Source: CAD feature listing. Evaluate the final solid. Frame: model axes, mm. Face numbers are marked on the shaded views. A direction names the side the tool comes from. Round coordinates to 2 decimals unless told otherwise and drop trailing zeros. Loops run counter-clockwise (first coordinate to the right, second up) from the corner with the lowest first, then second, coordinate; pieces in that order, holes last.
(1) Material intervals for probe 1 along X at (y, z) = (-3.25, 0.75); probe 2 along Z at (x, y) = (1.5, 2.75); probe 3 along X at (y, z) = (2.75, 3.5), sorted ascending.
(2) Section C-C, the plane x = 0. Return the cut outline in (y, z).
(3) Mould query, pull axis X, two halves, no side actions, for the marked faces 4 and 5. Classes: pulls with the +X half, pulls with the -X half, needs draft (parallel to the pull), parting line crosses it, or undercut.
(4) First-contact query: pin 1 Ø1 at (x, z) = (2.5, -3.5) entering from -Y; pin 2 Ø1.8 at (x, y) = (-2.5, 1.5) entering from -Z; pin 3 Ø2 at (x, z) = (-1.5, -3.5) entering from -Y. Flat tips, straight axial feed; report the tip coordinate or a pass-through.
(5) Section B-B, the plane y = 0. Return the cut outline in (x, z).
(6) Set-up query: the marked faces 1, 2 and 3. Return all of +Z, -Z, +X, -X, +Y, -Y with unobstructed straight access to the full face (end or side cutting, diameter ignored); none if empty.
```python
from build123d import *
from build123d import SkipClean  # not in build123d's __all__

# Parameters (mm, degrees)
F1_DEPTH     = 5
F2_DEPTH     = 5
F3_T3_DEPTH  = 12.521557359
F3_T6_ANGLE  = 198.0325102457
F3_T9_ANGLE  = 198.0325102457
F3_T12_DEPTH = 12.521557359
F3_T15_ANGLE = 209.516708524
F3_T18_DEPTH = 12.571682988
F3_T21_ANGLE = 144.0077008654
F3_T24_ANGLE = 53.9966137912
F3_T27_DEPTH = 7.0466201735
F3_T31_DEPTH = 8.0466201735


# Not quite as in the source:
# - a fillet or chamfer that OpenCascade refuses, or shapes differently, is made with other operations: its cross-section is extruded or revolved along the edge and cut away or added


with BuildPart() as f1:
    # F0 (on Top) → F1 (new body)
    with BuildSketch(Plane.XY):
        with BuildLine():
            ThreePointArc((-3.5355339059, -3.5355339059), (-2.1422777427, -4.5178143026), (-0.5, -4.9749371855))
            Line((-0.5, -4.9749371855), (-0.5, -0.5))
            Line((-0.5, -0.5), (-3.5355339059, -3.5355339059))
        make_face()
        with BuildLine():
            ThreePointArc((-0.5, -4.9749371855), (-0.2503138753, -4.9937303656), (0, -5))
            Line((0, -5), (0, 0))
            Line((0, 0), (-0.5, -0.5))
            Line((-0.5, -0.5), (-0.5, -4.9749371855))
        make_face()
        with BuildLine():
            ThreePointArc((0, -5), (0.2503138753, -4.9937303656), (0.5, -4.9749371855))
            Line((0.5, -4.9749371855), (0.5, 0.5))
            Line((0.5, 0.5), (0, 0))
            Line((0, 0), (0, -5))
        make_face()
        with BuildLine():
            ThreePointArc((0.5, -4.9749371855), (3.7080992435, -3.3541019662), (5, 0))
            ThreePointArc((5, 0), (4.6193976626, 1.9134171618), (3.5355339059, 3.5355339059))
            Line((3.5355339059, 3.5355339059), (0.5, 0.5))
            Line((0.5, 0.5), (0.5, -4.9749371855))
        make_face()
    extrude(amount=-F1_DEPTH)

    # F0 (on Top) → F2 (join)
    with BuildSketch(Plane.XY):
        with BuildLine():
            Line((-0.5, -0.5), (-0.5, 4.9749371855))
            ThreePointArc((-0.5, 4.9749371855), (-4.7093962486, 1.6797580105), (-3.5355339059, -3.5355339059))
            Line((-3.5355339059, -3.5355339059), (-0.5, -0.5))
        make_face()
        with BuildLine():
            Line((0.5, 0.5), (3.5355339059, 3.5355339059))
            ThreePointArc((3.5355339059, 3.5355339059), (2.1422777427, 4.5178143026), (0.5, 4.9749371855))
            Line((0.5, 4.9749371855), (0.5, 0.5))
        make_face()
        with BuildLine():
            ThreePointArc((0.5, -4.9749371855), (3.7080992435, -3.3541019662), (5, 0))
            ThreePointArc((5, 0), (4.6193976626, 1.9134171618), (3.5355339059, 3.5355339059))
            Line((3.5355339059, 3.5355339059), (0.5, 0.5))
            Line((0.5, 0.5), (0.5, -4.9749371855))
        make_face()
        with BuildLine():
            ThreePointArc((-3.5355339059, -3.5355339059), (-2.1422777427, -4.5178143026), (-0.5, -4.9749371855))
            Line((-0.5, -4.9749371855), (-0.5, -0.5))
            Line((-0.5, -0.5), (-3.5355339059, -3.5355339059))
        make_face()
    with SkipClean():  # cleaning this boolean's faces spoils the solid; the shape is the same uncleaned
        extrude(amount=F2_DEPTH)

    # F3: chamfer of 0.5 on 12 edges, made by hand


with BuildPart() as f3_tool1:
    # F3_s2 → F3_t3 (new body)
    with BuildSketch(Plane.XZ.offset(-6.2607786795)):
        Polygon((0.5, 4.5), (1, 5), (0.5, 5), align=None)
    extrude(amount=F3_T3_DEPTH)


with BuildPart() as f3_tool4:
    # F3_s5 → F3_t6 (revolve)
    with BuildSketch(Plane(origin=(0, 0, 0), x_dir=(0, 0, 1), z_dir=(-0.9876439195, 0.1567146713, 0))):
        Polygon((4.5, -5), (5, -4.5), (5, -5), align=None)
    revolve(axis=Axis((0, 0, 5), (0, 0, 1)), revolution_arc=F3_T6_ANGLE)


with BuildPart() as f3_tool7:
    # F3_s8 → F3_t9 (revolve)
    with BuildSketch(Plane(origin=(0, 0, 0), x_dir=(0, 0, 1), z_dir=(0.9876439195, -0.1567146713, 0))):
        Polygon((4.5, -5), (5, -4.5), (5, -5), align=None)
    revolve(axis=Axis((0, 0, 5), (0, 0, 1)), revolution_arc=F3_T9_ANGLE)


with BuildPart() as f3_tool10:
    # F3_s11 → F3_t12 (new body)
    with BuildSketch(Plane.XZ.offset(6.2607786795)):
        Polygon((-0.5, 4.5), (-1, 5), (-0.5, 5), align=None)
    extrude(amount=-F3_T12_DEPTH)


with BuildPart() as f3_tool13:
    # F3_s14 → F3_t15 (revolve)
    with BuildSketch(Plane(origin=(0, 0, 0), x_dir=(0, 0, 1), z_dir=(-0.5036480164, 0.863908951, 0))):
        Polygon((-4.5, -5), (-5, -4.5), (-5, -5), align=None)
    revolve(axis=Axis((0, 0, -5), (0, 0, 1)), revolution_arc=F3_T15_ANGLE)


with BuildPart() as f3_tool16:
    # F3_s17 → F3_t18 (new body)
    with BuildSketch(Plane(origin=(4.4447611459, 4.4447611459, 0), x_dir=(0, 0, 1), z_dir=(-0.7071067812, -0.7071067812, 0))):
        Polygon((-4.5, 0), (-5, -0.5), (-5, 0), align=None)
    extrude(amount=F3_T18_DEPTH)


with BuildPart() as f3_tool19:
    # F3_s20 → F3_t21 (revolve)
    with BuildSketch(Plane(origin=(0, 0, 0), x_dir=(0, 0, 1), z_dir=(0.987667306, -0.1565672143, 0))):
        Polygon((0.5, -5), (0, -4.5), (0, -5), align=None)
    revolve(axis=Axis((0, 0, 0), (0, 0, 1)), revolution_arc=F3_T21_ANGLE)


with BuildPart() as f3_tool22:
    # F3_s23 → F3_t24 (revolve)
    with BuildSketch(Plane(origin=(0, 0, 0), x_dir=(0, 0, 1), z_dir=(0.7071067812, -0.7071067812, 0))):
        Polygon((0.5, -5), (0, -4.5), (0, -5), align=None)
    revolve(axis=Axis((0, 0, 0), (0, 0, 1)), revolution_arc=F3_T24_ANGLE)


with BuildPart() as f3_tool25:
    # F3_s26 → F3_t27 (new body)
    with BuildSketch(Plane.XZ.offset(-6.2607786795)):
        Polygon((1, 0), (0.5, 0.5), (0.5, 0), align=None)
    extrude(amount=F3_T27_DEPTH)

    split(bisect_by=Plane(origin=(0, 0, 0), x_dir=(0, 0, 1), z_dir=(-0.7071067812, 0.7071067812, 0)), keep=Keep.TOP)


with BuildPart() as f3_tool29:
    # F3_s30 → F3_t31 (new body)
    with BuildSketch(Plane.XZ.offset(1.785841494)):
        Polygon((-1, 0), (-0.5, 0.5), (-0.5, 0), align=None)
    extrude(amount=-F3_T31_DEPTH)

    split(bisect_by=Plane(origin=(0, 0, 0), x_dir=(0, 0, 1), z_dir=(-0.7071067812, 0.7071067812, 0)), keep=Keep.TOP)


with BuildPart() as f1_1:
    add(f1.part, clean=False)

    # F3_t33: cut F3_tool1, F3_tool4, F3_tool7, F3_tool10, F3_tool13, F3_tool16, F3_tool19, F3_tool22, F3_tool25, F3_tool29
    add([f3_tool1.part, f3_tool4.part, f3_tool7.part, f3_tool10.part, f3_tool13.part, f3_tool16.part, f3_tool19.part, f3_tool22.part, f3_tool25.part, f3_tool29.part], mode=Mode.SUBTRACT)


solid = f1_1.part
```
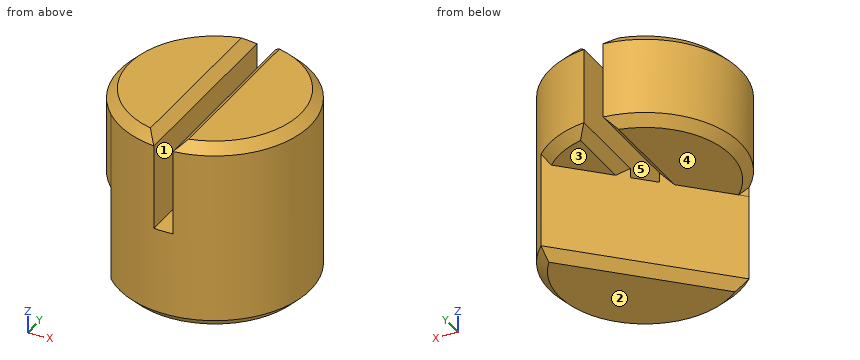
Output values:
1. probe 1: x = -3.8 to -0.5, 0.5 to 3.8
1. probe 2: z = 0 to 5
1. probe 3: x = -4.18 to -0.5, 0.5 to 4.18
2. outline: (-5, -4.5) - (-4.5, -5) - (-0.71, -5) - (0, -4.5) - (0, 0) - (-5, 0) - close
3. face 4: needs draft
3. face 5: undercut
4. pin 1: stops at y = -4.58
4. pin 2: stops at z = 0
4. pin 3: stops at y = -4.97
5. outline: (-5, 0.5) - (-4.5, 0) - (-1, 0) - (-0.5, 0.5) - (-0.5, 4.5) - (-1, 5) - (-4.5, 5) - (-5, 4.5) - close; (0, -4.5) - (0.71, -5) - (4.5, -5) - (5, -4.5) - (5, 4.5) - (4.5, 5) - (1, 5) - (0.5, 4.5) - (0.5, 0) - (0, 0) - close
6. face 1: +Z, +Y, -Y
6. face 2: -Z, +X, -X, +Y, -Y
6. face 3: -Z, -X, +Y
